from build123d import *

# Parameters (mm, degrees)
F1_DEPTH = 82
F2_R     = 5.5
F3_DEPTH = 20.001
F5_DEPTH = 20.001


with BuildPart() as f1:
    # F0 (on Front) → F1 (new body)
    with BuildSketch(Plane.XZ):
        with BuildLine():
            Line((0, 16), (0, 0))
            Line((0, 0), (38, 0))
            Line((38, 0), (38, -4))
            Line((38, -4), (98, -4))
            Line((98, -4), (98, 0))
            Line((98, 0), (136, 0))
            Line((136, 0), (136, 16))
            Line((136, 16), (92, 16))
            ThreePointArc((92, 16), (91.621063, 13.267949), (89.171573, 12))
            Line((89.171573, 12), (46.828427, 12))
            ThreePointArc((46.828427, 12), (44.378937, 13.267949), (44, 16))
            Line((44, 16), (0, 16))
        make_face()
    extrude(amount=F1_DEPTH)

    # F2 (on face) → F3 (cut, through all)
    with BuildSketch(Plane.XY.offset(16)):
        with Locations((14, -14)):
            Circle(F2_R)
        with Locations((14, -68)):
            Circle(F2_R)
        with Locations((122, -14)):
            Circle(F2_R)
        with Locations((122, -68)):
            Circle(F2_R)
    extrude(amount=-F3_DEPTH, mode=Mode.SUBTRACT)

    # F4 (on face) → F5 (cut, through all)
    with BuildSketch(Plane.XY.offset(16)):
        with BuildLine():
            Line((14, 0), (0, 0))
            Line((0, 0), (0, -14))
            ThreePointArc((0, -14), (4.100505, -4.100505), (14, 0))
        make_face()
        with BuildLine():
            Line((0, -68), (0, -82))
            Line((0, -82), (14, -82))
            ThreePointArc((14, -82), (4.100505, -77.899495), (0, -68))
        make_face()
        with BuildLine():
            Line((136, 0), (122, 0))
            ThreePointArc((122, 0), (131.899495, -4.100505), (136, -14))
            Line((136, -14), (136, 0))
        make_face()
        with BuildLine():
            Line((136, -82), (136, -68))
            ThreePointArc((136, -68), (131.899495, -77.899495), (122, -82))
            Line((122, -82), (136, -82))
        make_face()
    extrude(amount=-F5_DEPTH, mode=Mode.SUBTRACT)


solid = f1.part
The listing builds one solid part. Answer for the finished solid, in the listing's coordinates (mm). A direction names the side the tool comes from. Give positions to 0.01 mm unless a question says otherwise; leave off trailing zeros. Write each loop counter-clockwise with the first axis right and the second up, starting at its lowest first coordinate (ties: lowest second). Pieces come first, ordered by that corner, then holes. Notation, with made-up numbers: (70.25, 74) -> (104.25, 74) arc R19 ccw to (104.25, 102) -> close; hole circle Ø8 at (57, 57). An arc over 180 degrees is marked (long way). Use a Markdown table: item, result.
(1) Section C-C, the plane y = -16 is taken. Determine the outline of the cut face in (x, z), then the cut area to 3 significant figures.
Return value:
| item | result |
|---|---|
| outline | (0, 0) -> (8.88, 0) -> (8.88, 16) -> (0, 16) -> close; (19.12, 0) -> (38, 0) -> (38, -4) -> (98, -4) -> (98, 0) -> (116.88, 0) -> (116.88, 16) -> (92, 16) arc R3 cw to (89.17, 12) -> (46.83, 12) arc R3 cw to (44, 16) -> (19.12, 16) -> close; (127.12, 0) -> (136, 0) -> (136, 16) -> (127.12, 16) -> close |
| area | 1,900 mm2 |
(2) Section B-B, the plane z = 10.5 is taken. Determine the outline of the cut face in (x, y), then the cut area to 3 significant figures.
Return value:
| item | result |
|---|---|
| outline | (0, -68) arc R14 ccw to (14, -82) -> (122, -82) arc R14 ccw to (136, -68) -> (136, -14) arc R14 ccw to (122, 0) -> (14, 0) arc R14 ccw to (0, -14) -> close; hole circle Ø11 at (14, -68); hole circle Ø11 at (14, -14); hole circle Ø11 at (122, -68); hole circle Ø11 at (122, -14) |
| area | 10,600 mm2 |
(3) Section A-A, the plane y = -28 is taken. Determine the outline of the cut face in (x, z).
Return value:
| item | result |
|---|---|
| outline | (0, 0) -> (38, 0) -> (38, -4) -> (98, -4) -> (98, 0) -> (136, 0) -> (136, 16) -> (92, 16) arc R3 cw to (89.17, 12) -> (46.83, 12) arc R3 cw to (44, 16) -> (0, 16) -> close |
(4) Section D-D, the plane x = 107 is taken. Determine the outline of the cut face in (y, z), then the cut area to 3 significant figures.
Return value:
| item | result |
|---|---|
| outline | (-82, 0) -> (0, 0) -> (0, 16) -> (-82, 16) -> close |
| area | 1,310 mm2 |
(5) Determine the mould class of faces 1 (the flat face through (68, -40, 12)), 2 (the flat face through (114, -40, 16)), 3 (the flat face through (0, -41, 8)) for opening direction X: released by +X, released by -X, zero draft, split by the parting line, or undercut.
Return value:
| item | result |
|---|---|
| face 1 | undercut |
| face 2 | zero draft |
| face 3 | released by -X |
(6) Flat-ended cylindrical pins translate along their axes: P1, Ø10, axis at x = 116, y = -44.5, coming from the -Z side; P2, Ø2, axis at y = -60, z = -2, coming from the -X side; P3, Ø2, axis at y = -55.5, z = -2.5, coming from the +X side. Find the tip coordinate at first contact, or state that the pin passes through.
Return value:
| item | result |
|---|---|
| P1 | z = 0 |
| P2 | x = 38 |
| P3 | x = 98 |
(7) Find the intervals of material crossed by probe 1 along Y at (x, z) = (14, 3); probe 2 along Y at (x, z) = (15, 8); probe 3 along Z at (x, y) = (29.5, -15), in increasing order. Write a range as from..to.
Return value:
| item | result |
|---|---|
| probe 1 | -82..-73.5, -62.5..-19.5, -8.5..0 |
| probe 2 | -82..-73.41, -62.59..-19.41, -8.59..0 |
| probe 3 | 0..16 |
(8) For faces 4 (the cylindrical face through (132, -77.8, 8.1)), 5 (the flat face through (117, -40, 0)), 6 (the cylindrical face through (44.4, -40.43, 13.24)), 7 (the cylindrical face through (116.505, -13.758, 8.112)), 8 (the flat face through (38, -40, -2)), determine the directions among +Z, -Z, +X, -X, +Y, -Y from which every point of the face is accessible in a straight line to the end or side of a thin tool.
Return value:
| item | result |
|---|---|
| face 4 | +Z, -Z, +X, -Y |
| face 5 | -Z, +X, +Y, -Y |
| face 6 | +Y, -Y |
| face 7 | +Z, -Z |
| face 8 | -Z, -X, +Y, -Y |
